```python
from build123d import *

# Parameters (mm, degrees)
SKETCH1_R             = 7.5
SKETCH1_R_2           = 2.5
SKETCH1_W             = 2
SKETCH1_H             = 5
BOSS_EXTRUDE1_DEPTH   = 7.5
CUT_EXTRUDE1_START    = 7.5
SKETCH2_W             = 36
SKETCH2_H             = 11
CUT_EXTRUDE1_DEPTH    = 12
SKETCH3_W             = 1.5
SKETCH3_H             = 2.5
SKETCH3_W_2           = 10
SKETCH3_H_2           = 7
CUT_EXTRUDE2_DEPTH    = 40
SKETCH5_W             = 1
SKETCH5_H             = 12
CUT_EXTRUDE3_DEPTH    = 20
BOSS_EXTRUDE2_START   = 14
SKETCH6_W             = 3
SKETCH6_H             = 0.5
BOSS_EXTRUDE2_DEPTH   = 5
FILLET2_R             = 1.5
LPATTERN4_START       = -12
LPATTERN4_OUTLINE_W   = 2
LPATTERN4_OUTLINE_H   = 12
LPATTERN4_DEPTH       = 1
LPATTERN4_START_2     = -6
LPATTERN4_2_OUTLINE_W = 2
LPATTERN4_2_OUTLINE_H = 12
LPATTERN4_2_DEPTH     = 1
LPATTERN4_START_3     = -11
LPATTERN4_3_DEPTH     = 5
LPATTERN4_4_DEPTH     = 5
BOSS_EXTRUDE3_START   = -4.5
BOSS_EXTRUDE3_DEPTH   = 8
SKETCH8_W             = 3
SKETCH8_H             = 4
CUT_EXTRUDE4_DEPTH    = 3


# Read off the part's stored shape, not the designer's step: LPattern4
with BuildPart() as part:
    # Sketch1 → Boss-Extrude1 (new, symmetric)
    # profile 1 of 4: a face of its own
    with BuildSketch(Plane(origin=(0, 0, 0), x_dir=(1, 0, 0), z_dir=(0, 1, 0))):
        with BuildLine():
            ThreePointArc((20, -7.5), (12.5, 0), (20, 7.5))
            Line((20, 7.5), (-20, 7.5))
            ThreePointArc((-20, 7.5), (-23.535533906, 6.035533906), (-25, 2.5))
            Line((-25, 2.5), (-25, -2.5))
            ThreePointArc((-25, -2.5), (-23.535533906, -6.035533906), (-20, -7.5))
            Line((-20, -7.5), (20, -7.5))
        make_face()
    # profile 2 of 4: a face of its own
    with BuildSketch(Plane(origin=(0, 0, 0), x_dir=(1, 0, 0), z_dir=(0, 1, 0))):
        with Locations((20, 0)):
            Circle(SKETCH1_R)
        with Locations(Location((20, 0, 0), (0, 0, 270))):
            Circle(SKETCH1_R_2, mode=Mode.SUBTRACT)
    # profile 3 of 4: a face of its own
    with BuildSketch(Plane(origin=(0, 0, 0), x_dir=(1, 0, 0), z_dir=(0, 1, 0))):
        with BuildLine():
            Line((27.5, 2.5), (27.5, 7.5))
            Line((27.5, 7.5), (20, 7.5))
            ThreePointArc((20, 7.5), (25.303300859, 5.303300859), (27.5, 0))
            Line((27.5, 0), (27.5, 2.5))
        make_face()
    # profile 4 of 4: a face of its own
    with BuildSketch(Plane(origin=(0, 0, 0), x_dir=(1, 0, 0), z_dir=(0, 1, 0))):
        with Locations((28.5, 5)):
            Rectangle(SKETCH1_W, SKETCH1_H)
    extrude(amount=BOSS_EXTRUDE1_DEPTH, both=True)

    # Sketch2 → Cut-Extrude1 (cut)
    with BuildSketch(Plane.XY.offset(CUT_EXTRUDE1_START)):
        Rectangle(SKETCH2_W, SKETCH2_H)
    extrude(amount=-CUT_EXTRUDE1_DEPTH, mode=Mode.SUBTRACT)

    # Sketch3 → Cut-Extrude2 (cut)
    with BuildSketch(Plane(origin=(0, 0, 0), x_dir=(0, 0, -1), z_dir=(1, 0, 0))):
        with Locations((-6.75, 0)):
            Rectangle(SKETCH3_W, SKETCH3_H)
        with Locations((-1, 0)):
            Rectangle(SKETCH3_W_2, SKETCH3_H_2)
    extrude(amount=CUT_EXTRUDE2_DEPTH, mode=Mode.SUBTRACT)

    # Sketch5 → Cut-Extrude3 (cut, symmetric)
    with BuildSketch(Plane(origin=(0, 0, 0), x_dir=(1, 0, 0), z_dir=(0, 1, 0))):
        with Locations((8.5, -1.5)):
            Rectangle(SKETCH5_W, SKETCH5_H)
        with Locations((14.5, -1.5)):
            Rectangle(SKETCH5_W, SKETCH5_H)
    extrude(amount=CUT_EXTRUDE3_DEPTH, both=True, mode=Mode.SUBTRACT)

    # Sketch6 → Boss-Extrude2 (add)
    with BuildSketch(Plane(origin=(0, 0, 0), x_dir=(0, 0, -1), z_dir=(1, 0, 0)).offset(BOSS_EXTRUDE2_START)):
        with Locations((-6, 5.25)):
            Rectangle(SKETCH6_W, SKETCH6_H)
        with Locations((-6, -5.25)):
            Rectangle(SKETCH6_W, SKETCH6_H)
    extrude(amount=-BOSS_EXTRUDE2_DEPTH)

    # Fillet2
    # the kernel refuses this fillet: 1.5 mm, written as the material it takes off along each edge
    with BuildSketch(Plane(origin=(16.795084972, 5, 4.5), x_dir=(0, 0, 1), z_dir=(-1, 0, 0))) as fillet2_piece_1:
        with BuildLine():
            CenterArc((1.118033989, 1.5), FILLET2_R, 221.810314896, 48.189685104)
            Line((0, 0.5), (0, 0))
            Line((0, 0), (1.118033989, 0))
        make_face()
    extrude(amount=10.590169944, mode=Mode.SUBTRACT)
    with BuildSketch(Plane(origin=(17.75, 5, 7.5), x_dir=(0, 1, 0), z_dir=(-1, 0, 0))) as fillet2_piece_2_section:
        with BuildLine():
            CenterArc((FILLET2_R, FILLET2_R), FILLET2_R, 180, 90)
            Line((0, FILLET2_R), (0, 0))
            Line((0, 0), (FILLET2_R, 0))
        make_face()
    fillet2_piece_2 = extrude(amount=12.5, mode=Mode.PRIVATE)
    fillet2_piece_2 = split(fillet2_piece_2, bisect_by=Plane(origin=(15, 5.743185978, 7.388433108), z_dir=(-1, 0, 0)), keep=Keep.TOP, mode=Mode.PRIVATE)
    fillet2_piece_2 = split(fillet2_piece_2, bisect_by=Plane(origin=(8, 5.743185978, 7.388433108), z_dir=(1, 0, 0)), keep=Keep.TOP, mode=Mode.PRIVATE)
    add(fillet2_piece_2, mode=Mode.SUBTRACT)
    with BuildSketch(Plane(origin=(16.795084972, -5, 4.5), x_dir=(0, 0, 1), z_dir=(-1, 0, 0))) as fillet2_piece_3:
        with BuildLine():
            CenterArc((1.118033989, -1.5), FILLET2_R, 90, 48.189685104)
            Line((0, -0.5), (0, 0))
            Line((0, 0), (1.118033989, 0))
        make_face()
    extrude(amount=10.590169944, mode=Mode.SUBTRACT)
    with BuildSketch(Plane(origin=(17.75, -5, 7.5), x_dir=(0, -1, 0), z_dir=(-1, 0, 0))) as fillet2_piece_4_section:
        with BuildLine():
            CenterArc((FILLET2_R, -FILLET2_R), FILLET2_R, 90, 90)
            Line((0, -FILLET2_R), (0, 0))
            Line((0, 0), (FILLET2_R, 0))
        make_face()
    fillet2_piece_4 = extrude(amount=8.75, mode=Mode.PRIVATE)
    fillet2_piece_4 = split(fillet2_piece_4, bisect_by=Plane(origin=(15, -5.743185978, 7.388433108), z_dir=(-1, 0, 0)), keep=Keep.TOP, mode=Mode.PRIVATE)
    add(fillet2_piece_4, mode=Mode.SUBTRACT)

    # LPattern4 outline → LPattern4 (cut)
    with BuildSketch(Plane.YZ.offset(LPATTERN4_START)):
        with Locations((-6.5, 1.5)):
            Rectangle(LPATTERN4_OUTLINE_W, LPATTERN4_OUTLINE_H)
        with Locations((6.5, 1.5)):
            Rectangle(LPATTERN4_OUTLINE_W, LPATTERN4_OUTLINE_H)
    extrude(amount=LPATTERN4_DEPTH, mode=Mode.SUBTRACT)

    # LPattern4 2 outline → LPattern4 2 (cut)
    with BuildSketch(Plane.YZ.offset(LPATTERN4_START_2)):
        with Locations((-6.5, 1.5)):
            Rectangle(LPATTERN4_2_OUTLINE_W, LPATTERN4_2_OUTLINE_H)
        with Locations((6.5, 1.5)):
            Rectangle(LPATTERN4_2_OUTLINE_W, LPATTERN4_2_OUTLINE_H)
    extrude(amount=LPATTERN4_2_DEPTH, mode=Mode.SUBTRACT)

    # LPattern4 3 outline → LPattern4 3 (cut)
    with BuildSketch(Plane.YZ.offset(LPATTERN4_START_3)):
        with BuildLine():
            ThreePointArc((-6.5, 7.5), (-5.964766865, 7.401258539), (-5.5, 7.118033989))
            Line((-5.5, 7.118033989), (-5.5, 7.5))
            Line((-5.5, 7.5), (-6.5, 7.5))
        make_face()
        with BuildLine():
            Line((6.5, 7.5), (5.5, 7.5))
            Line((5.5, 7.5), (5.5, 7.118033989))
            ThreePointArc((5.5, 7.118033989), (5.964766865, 7.401258539), (6.5, 7.5))
        make_face()
    extrude(amount=LPATTERN4_3_DEPTH, mode=Mode.SUBTRACT)

    # LPattern4 4 outline → LPattern4 4 (add)
    with BuildSketch(Plane.YZ.offset(LPATTERN4_START_3)):
        with BuildLine():
            Line((-5, 5.618033989), (-5, 6))
            ThreePointArc((-5, 6), (-5.130693606, 6.612372436), (-5.5, 7.118033989))
            Line((-5.5, 7.118033989), (-5.5, 4.5))
            ThreePointArc((-5.5, 4.5), (-5.130693606, 5.005661553), (-5, 5.618033989))
        make_face()
        with BuildLine():
            Line((5.5, 4.5), (5.5, 7.118033989))
            ThreePointArc((5.5, 7.118033989), (5.130693606, 6.612372436), (5, 6))
            Line((5, 6), (5, 5.618033989))
            ThreePointArc((5, 5.618033989), (5.130693606, 5.005661553), (5.5, 4.5))
        make_face()
    extrude(amount=LPATTERN4_4_DEPTH)

    # Sketch7 → Boss-Extrude3 (add)
    with BuildSketch(Plane.XY.offset(BOSS_EXTRUDE3_START)):
        with BuildLine():
            Line((4, -1.5), (-4, -1.5))
            ThreePointArc((-4, -1.5), (-4.707106781, -1.207106781), (-5, -0.5))
            Line((-5, -0.5), (-5, 0.5))
            ThreePointArc((-5, 0.5), (-4.707106781, 1.207106781), (-4, 1.5))
            Line((-4, 1.5), (4, 1.5))
            ThreePointArc((4, 1.5), (4.707106781, 1.207106781), (5, 0.5))
            Line((5, 0.5), (5, -0.5))
            ThreePointArc((5, -0.5), (4.707106781, -1.207106781), (4, -1.5))
        make_face()
    extrude(amount=BOSS_EXTRUDE3_DEPTH)

    # Sketch8 → Cut-Extrude4 (cut)
    with BuildSketch(Plane.ZY.offset(5)):
        Rectangle(SKETCH8_W, SKETCH8_H)
    extrude(amount=-CUT_EXTRUDE4_DEPTH, mode=Mode.SUBTRACT)


solid = part.part
```
Here's how the part is built. I have some questions about the finished solid (model axes, mm). A direction names the side the tool comes from. Give positions to 0.01 mm unless a question says otherwise; leave off trailing zeros. Order: outer loops, then holes, each group sorted by start corner. A loop starts at its lowest first (then second) coordinate and runs counter-clockwise, first axis right, second up. Notation, with made-up numbers: M 9.5,-26 L 66.5,-26 A19 cw 66.5,-11 Z; hole C 38.25,18.25 d4. An arc over 180 degrees is marked long. Use a Markdown table: item, result. Add a question column.
1. Suppose I cut it at A-A (x = -3.5). List the corners of the cut face in (y, z) for me, and give its area (3 significant figures).
2. Suppose I cut it at C-C (y = -2.25). List the corners of the cut face in (x, z) for me.
3. If we mould it in two halves opening along Y, with no side actions, what happens to faces 1 (the flat face through (12, 7, 7.5)), 2 (the cylindrical face through (11.54, -5.45, 7.07))? For each: +Y half, -Y half, draft (parallel to the pull), parting line (faces both ways), or undercut.
4. I need wall thicknesses on probe 1 along Y at (x, z) = (3, -1.5); probe 2 along X at (y, z) = (-6.25, 0); probe 3 along X at (y, z) = (-4.85, 0). Which ranges of each line are inside material? Lowest first, please. Write a range as from..to.
5. For pin 1 Ø0.9 at (x, y) = (-1, 0.5) entering from +Z; pin 2 Ø1.6 at (y, z) = (6.5, 4.5) entering from +X; pin 3 Ø0.5 at (y, z) = (0, 0) entering from +X, each with a flat end and sliding along its axis, tell me the tip position at first contact or that it passes through.
6. Suppose I cut it at D-D (z = -3). Give the number of separate pieces and of enclosed holes in the cut face, and give its area (3 significant figures).
7. Suppose I cut it at B-B (y = 4.5). List the corners of the cut face in (x, z) for me, and give its area (3 significant figures).
8. On a 3-axis mill with a long thin cutter (end or side, diameter ignored), from which of +Z, -Z, +X, -X, +Y, -Y can I reach the whole of each face in a straight line? I mean faces 3 (the cylindrical face through (-8.535, -5.134, 4.998)), 4 (the flat face through (27.5, 6, -1)), 5 (the flat face through (-6, 7, 2)). Say none if no direction works.
Results list:
| question | item | result |
|---|---|---|
| 1 | outline | M -7.5,-7.5 L 7.5,-7.5 L 7.5,7.5 L 5.5,7.5 L 5.5,-4.5 L 1.5,-4.5 L 1.5,-1.5 L -1.5,-1.5 L -1.5,-4.5 L -5.5,-4.5 L -5.5,7.5 L -7.5,7.5 Z; M -1.5,1.5 L 1.5,1.5 L 1.5,3.5 L -1.5,3.5 Z |
| 1 | area | 108 mm² |
| 2 | outline | M -25,-2.5 A5 ccw -20,-7.5 L 29.5,-7.5 L 29.5,-4 L 18,-4 L 18,-4.5 L -18,-4.5 L -18,7.5 L -20,7.5 A5 ccw -25,2.5 Z; M 18,6 L 24.5,6 A7.5 ccw 20,7.5 L 18,7.5 Z |
| 3 | face 1 | draft |
| 3 | face 2 | undercut |
| 4 | probe 1 | y = -7.5..-5.5, -1.5..1.5, 5.5..7.5 |
| 4 | probe 2 | x = -25..-12, -11..-6, -5..8, 9..14, 15..17.5, 22.5..27.5 |
| 4 | probe 3 | x = -25..-18, 22.5..27.5 |
| 5 | pin 1 | stops at z = 3.5 |
| 5 | pin 2 | stops at x = 26.52 |
| 5 | pin 3 | stops at x = 5 |
| 6 | separate pieces | 10 |
| 6 | enclosed holes | 0 |
| 6 | area | 354 mm² |
| 7 | outline | M -25,-2.5 A5 ccw -20,-7.5 L 29.5,-7.5 L 29.5,-2.5 L 27.5,-2.5 L 27.5,0 A7.5 ccw 20,7.5 L 18,7.5 L 18,1.5 A2.5 cw long 18,-1.5 L 18,-4.5 L -18,-4.5 L -18,7.5 L -20,7.5 A5 ccw -25,2.5 Z |
| 7 | area | 324 mm² |
| 8 | face 3 | none |
| 8 | face 4 | +Z, +X, +Y, -Y |
| 8 | face 5 | +Z, +Y, -Y |
